```python
from build123d import *

# Parameters (mm, degrees)
SM_BASE_FLANGE_1_DEPTH = 400
SKETCH_8_R             = 2.3
CUT_EXTRUDE_2_DEPTH    = 598.920738894
SKETCH_9_R             = 2.3
CUT_EXTRUDE_3_DEPTH    = 10
CHAMFER_1_SIZE         = 2.05


# Sheet-metal steps are written as plain solids
with BuildPart() as part:
    # Sketch 1 → Базовая кромка1 (new body)
    with BuildSketch(Plane.XY):
        with BuildLine():
            Line((0, 0), (0, 82.1))
            ThreePointArc((0, 82.1), (-1.171572875, 84.928427125), (-4, 86.1))
            Line((-4, 86.1), (-432, 86.1))
            ThreePointArc((-432, 86.1), (-434.828427125, 84.928427125), (-436, 82.1))
            Line((-436, 82.1), (-436, 0))
            Line((-436, 0), (-434, 0))
            Line((-434, 0), (-434, 82.1))
            ThreePointArc((-434, 82.1), (-433.414213562, 83.514213562), (-432, 84.1))
            Line((-432, 84.1), (-4, 84.1))
            ThreePointArc((-4, 84.1), (-2.585786438, 83.514213562), (-2, 82.1))
            Line((-2, 82.1), (-2, 0))
            Line((-2, 0), (0, 0))
        make_face()
    extrude(amount=SM_BASE_FLANGE_1_DEPTH)

    # Эскиз8 → Вырез-Вытянуть2 (cut, through all)
    with BuildSketch(Plane(origin=(0, 0, 0), x_dir=(0, 0, -1), z_dir=(1, 0, 0))):
        with Locations(Location((-373, 8, 0), (0, 0, 90))):
            Circle(SKETCH_8_R)
        with Locations(Location((-200, 8, 0), (0, 0, 90))):
            Circle(SKETCH_8_R)
        with Locations(Location((-27, 8, 0), (0, 0, 90))):
            Circle(SKETCH_8_R)
    extrude(amount=-CUT_EXTRUDE_2_DEPTH, mode=Mode.SUBTRACT)

    # Эскиз9 → Вырез-Вытянуть3 (cut)
    with BuildSketch(Plane(origin=(0, 86.1, 0), x_dir=(1, 0, 0), z_dir=(0, 1, 0))):
        with Locations(Location((-42, -392, 0), (0, 0, 180))):
            Circle(SKETCH_9_R)
        with Locations(Location((-394, -392, 0), (0, 0, 180))):
            Circle(SKETCH_9_R)
        with Locations(Location((-42, -8, 0), (0, 0, 180))):
            Circle(SKETCH_9_R)
        with Locations(Location((-394, -8, 0), (0, 0, 180))):
            Circle(SKETCH_9_R)
    extrude(amount=-CUT_EXTRUDE_3_DEPTH, mode=Mode.SUBTRACT)

    # Фаска1
    # the kernel refuses this chamfer: 2.05 mm, written as the material it takes off along each edge
    with BuildSketch(Plane(origin=(-436, 8, 373), x_dir=(0, 1, 0), z_dir=(0, 0, -1))) as chamfer_1_piece_1:
        Polygon((2.3 + CHAMFER_1_SIZE, 0), (2.3, CHAMFER_1_SIZE), (2.3, 0), align=None)
    revolve(axis=Axis((-436, 8, 373), (1, 0, 0)), mode=Mode.SUBTRACT)
    with BuildSketch(Plane(origin=(0, 8, 373), x_dir=(0, 1, 0), z_dir=(0, 0, -1))) as chamfer_1_piece_2:
        Polygon((2.3, -CHAMFER_1_SIZE), (2.3 + CHAMFER_1_SIZE, 0), (2.3, 0), align=None)
    revolve(axis=Axis((0, 8, 373), (1, 0, 0)), mode=Mode.SUBTRACT)
    with BuildSketch(Plane(origin=(-436, 8, 200), x_dir=(0, 1, 0), z_dir=(0, 0, -1))) as chamfer_1_piece_3:
        Polygon((2.3 + CHAMFER_1_SIZE, 0), (2.3, CHAMFER_1_SIZE), (2.3, 0), align=None)
    revolve(axis=Axis((-436, 8, 200), (1, 0, 0)), mode=Mode.SUBTRACT)
    with BuildSketch(Plane(origin=(0, 8, 200), x_dir=(0, 1, 0), z_dir=(0, 0, -1))) as chamfer_1_piece_4:
        Polygon((2.3, -CHAMFER_1_SIZE), (2.3 + CHAMFER_1_SIZE, 0), (2.3, 0), align=None)
    revolve(axis=Axis((0, 8, 200), (1, 0, 0)), mode=Mode.SUBTRACT)
    with BuildSketch(Plane(origin=(-436, 8, 27), x_dir=(0, 1, 0), z_dir=(0, 0, -1))) as chamfer_1_piece_5:
        Polygon((2.3 + CHAMFER_1_SIZE, 0), (2.3, CHAMFER_1_SIZE), (2.3, 0), align=None)
    revolve(axis=Axis((-436, 8, 27), (1, 0, 0)), mode=Mode.SUBTRACT)
    with BuildSketch(Plane(origin=(0, 8, 27), x_dir=(0, 1, 0), z_dir=(0, 0, -1))) as chamfer_1_piece_6:
        Polygon((2.3, -CHAMFER_1_SIZE), (2.3 + CHAMFER_1_SIZE, 0), (2.3, 0), align=None)
    revolve(axis=Axis((0, 8, 27), (1, 0, 0)), mode=Mode.SUBTRACT)
    with BuildSketch(Plane(origin=(-42, 86.1, 392), x_dir=(-1, 0, 0), z_dir=(0, 0, -1))) as chamfer_1_piece_7:
        Polygon((2.3, -CHAMFER_1_SIZE), (2.3 + CHAMFER_1_SIZE, 0), (2.3, 0), align=None)
    revolve(axis=Axis((-42, 86.1, 392), (0, 1, 0)), mode=Mode.SUBTRACT)
    with BuildSketch(Plane(origin=(-394, 86.1, 392), x_dir=(-1, 0, 0), z_dir=(0, 0, -1))) as chamfer_1_piece_8:
        Polygon((2.3, -CHAMFER_1_SIZE), (2.3 + CHAMFER_1_SIZE, 0), (2.3, 0), align=None)
    revolve(axis=Axis((-394, 86.1, 392), (0, 1, 0)), mode=Mode.SUBTRACT)
    with BuildSketch(Plane(origin=(-42, 86.1, 8), x_dir=(-1, 0, 0), z_dir=(0, 0, -1))) as chamfer_1_piece_9:
        Polygon((2.3, -CHAMFER_1_SIZE), (2.3 + CHAMFER_1_SIZE, 0), (2.3, 0), align=None)
    revolve(axis=Axis((-42, 86.1, 8), (0, 1, 0)), mode=Mode.SUBTRACT)
    with BuildSketch(Plane(origin=(-394, 86.1, 8), x_dir=(-1, 0, 0), z_dir=(0, 0, -1))) as chamfer_1_piece_10:
        Polygon((2.3, -CHAMFER_1_SIZE), (2.3 + CHAMFER_1_SIZE, 0), (2.3, 0), align=None)
    revolve(axis=Axis((-394, 86.1, 8), (0, 1, 0)), mode=Mode.SUBTRACT)


solid = part.part
```
Source: CAD feature listing. Evaluate the final solid. Frame: model axes, mm. A direction names the side the tool comes from. Coordinates: 2 decimals unless noted, no trailing zeros. Order: outer loops, then holes, each group sorted by start corner. A loop starts at its lowest first (then second) coordinate and runs counter-clockwise, first axis right, second up. Notation, with made-up numbers: M 38.25,72.5 L 68.25,72.5 A29 cw 68.25,111.5 Z; hole C 77.5,-40 d7. An arc over 180 degrees is marked long. Write each question's results on one line, items separated by ' | '. Start each with the question number.
1) Draft query along X for faces 3 (the face through (-436, 42, 197)), 4 (the face through (-221, 84.1, 197)), 5 (the face through (-219, 85, 400)). Return one class per face: released by +X, released by -X, zero draft, split by the parting line, or undercut.
2) Access query for faces 1 (the face through (-215, 86.1, 197)), 2 (the face through (-434, 40, 197)). Directions: +Z, -Z, +X, -X, +Y, -Y. A direction counts if a zero-diameter tool reaches every point of the face in a straight line with its end or side. Return the directions, or none.
3) Line query: line 1 (X direction, y = 30, z = 231.5); line 2 (Y direction, x = -399.5, z = 352). Output: solid intervals per line, ascending. Write a range as from..to.
4) Section query C-C (x = -278). Return the cut outline in (y, z).
5) Section query B-B (z = 340). Return the cut outline in (x, y), plus the area to 3 significant figures.
6) Section query A-A (y = 44.5). Return the cut outline in (x, z), plus the area to 3 significant figures.
Answers:
1) face 3: released by -X | face 4: undercut | face 5: zero draft
2) face 1: +Z, -Z, +X, -X, +Y | face 2: +Z, -Z, -Y
3) line 1: x = -436..-434, -2..0 | line 2: y = 84.1..86.1
4) outline: M 84.1,0 L 86.1,0 L 86.1,400 L 84.1,400 Z
5) outline: M -436,0 L -434,0 L -434,82.1 A2 cw -432,84.1 L -4,84.1 A2 cw -2,82.1 L -2,0 L 0,0 L 0,82.1 A4 ccw -4,86.1 L -432,86.1 A4 ccw -436,82.1 Z | area: 1,200 mm^2
6) outline: M -436,0 L -434,0 L -434,400 L -436,400 Z; M -2,0 L 0,0 L 0,400 L -2,400 Z | area: 1,600 mm^2
